from build123d import *

# Parameters (mm, degrees)
EXTRUDE_1_DEPTH = 5


with BuildPart() as part:
    # 草图2 → 凸台-拉伸1 (new body)
    with BuildSketch(Plane(origin=(0, 0, 0), x_dir=(0, 0, -1), z_dir=(1, 0, 0))):
        with BuildLine():
            Line((-7.45, 8), (7.45, 8))
            ThreePointArc((7.45, 8), (10, 5.45), (12.55, 8))
            Line((12.55, 8), (18, 8))
            Line((18, 8), (18, 0))
            Line((18, 0), (-18, 0))
            Line((-18, 0), (-18, 8))
            Line((-18, 8), (-12.55, 8))
            ThreePointArc((-12.55, 8), (-10, 5.45), (-7.45, 8))
        make_face()
    extrude(amount=EXTRUDE_1_DEPTH)


solid = part.part
Geometry check sheet. Reference: the model listing, model coordinates, mm. Round coordinates to 2 decimals unless told otherwise and drop trailing zeros. Loops run counter-clockwise (first coordinate to the right, second up) from the corner with the lowest first, then second, coordinate; pieces in that order, holes last.
Item 1: Cross-section at B-B on z = -10. Record the boundary of the cut face in (x, y), then the cut area to 4 significant figures.
Item 2: Mould release check, pull along Z, two halves, no side actions. Record for faces 1 (the flat face through (2, 4, -18)), 2 (the cylindrical face through (2.46, 5.45, 10.06)), 3 (the flat face through (2, 0, 0)): pulls with the +Z half, pulls with the -Z half, needs draft (parallel to the pull), parting line crosses it, or undercut.
Item 3: Cross-section at A-A on x = 2.9. Record the boundary of the cut face in (y, z).
Item 4: Thickness scan on line 1 (Z direction, x = 0.6, y = 5.75); line 2 (Z direction, x = 1.15, y = 7.25); line 3 (Y direction, x = 3.8, z = 10). Record the ranges inside material, lowest first.
Answer sheet:
1. outline: (0, 0) - (5, 0) - (5, 5.45) - (0, 5.45) - close
1. area: 27.25 mm2
2. face 1: pulls with the -Z half
2. face 2: undercut
2. face 3: needs draft
3. outline: (0, -18) - (8, -18) - (8, -12.55) arc R2.55 cw to (8, -7.45) - (8, 7.45) arc R2.55 cw to (8, 12.55) - (8, 18) - (0, 18) - close
4. line 1: z = -18 to -11.2, -8.8 to 8.8, 11.2 to 18
4. line 2: z = -18 to -12.44, -7.56 to 7.56, 12.44 to 18
4. line 3: y = 0 to 5.45
